Geometry check sheet. Reference: drawing and pictorial views, mm from the part's lowest x, y, z. Round coordinates to 2 decimals unless told otherwise and drop trailing zeros. Loops run counter-clockwise (first coordinate to the right, second up) from the corner with the lowest first, then second, coordinate; pieces in that order, holes last. Notation, with made-up numbers: (-26, 50) -> (4, 50) arc R20 ccw to (4, 64) -> close; hole circle Ø9 at (48, -12.75). An arc over 180 degrees is marked (long way). Use one line per item in the form item = value.
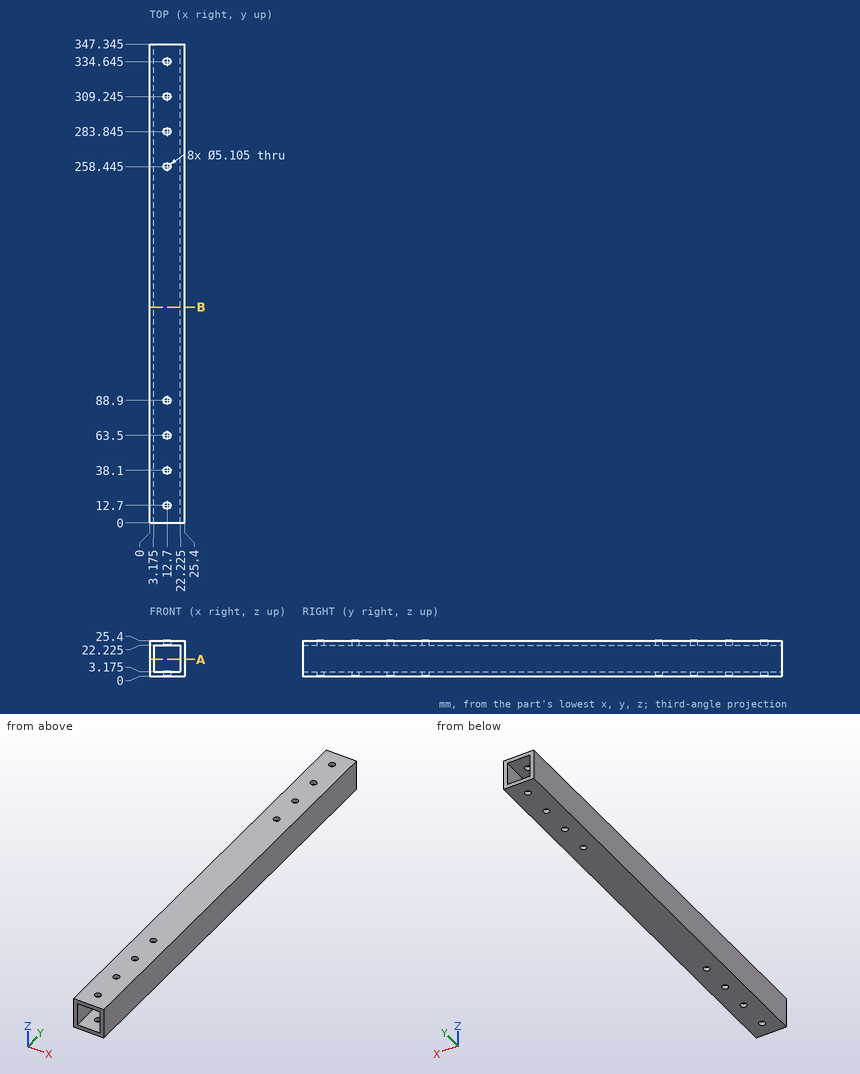
1. Section check B-B (y = 156.5). Record the boundary of the cut face in (x, z) (1 decimal).
Return value:
outline = (0, 0) -> (25.4, 0) -> (25.4, 25.4) -> (0, 25.4) -> close; hole (3.2, 3.2) -> (22.2, 3.2) -> (22.2, 22.2) -> (3.2, 22.2) -> close
2. Section check A-A (z = 12). Record the boundary of the cut face in (x, y) (1 decimal).
Return value:
outline = (0, 0) -> (3.2, 0) -> (3.2, 347.3) -> (0, 347.3) -> close; (22.2, 0) -> (25.4, 0) -> (25.4, 347.3) -> (22.2, 347.3) -> close
3. Material ranges on line 1 along Z through (x, y) = (19.5, 201.5) (1 decimal); line 2 along X through (y, z) = (88.9, 24.5), recorded low to high.
Return value:
line_1 = 0 to 3.2, 22.2 to 25.4
line_2 = 0 to 10.15, 15.25 to 25.4
4. Gauge pin test, flat ends, axial feed: pin 1 (4 mm diameter, centred on x = 12.7, y = 309.245, fed in from -Z); pin 2 (12 mm diameter, centred on x = 9.5, z = 20, fed in from -Y). Record the tip position at first contact, or that the pin passes through.
Return value:
pin_1 = through
pin_2 = 0
